The figure shows three views and two pictorial views of one solid part (mm, origin at its lowest corner). Answer the questions. A direction names the side the tool comes from. Coordinates: 2 decimals unless noted, no trailing zeros. Write each loop counter-clockwise with the first axis right and the second up, starting at its lowest first coordinate (ties: lowest second). Pieces come first, ordered by that corner, then holes.
Item 1: Section B-B (y = 112.5) is taken. Give the vertices of the cut face in (x, z), then the cut area to 3 significant figures.
Item 2: A tool of negligible diameter and unlimited length cuts with its end or side. For the marked faces 1 and 2, from which of +Z, -Z, +X, -X, +Y, -Y can it reach the whole face along a straight path? Write none if from no direction.
Item 3: Straight lines are drawn through the part: probe 1 along Y at (x, z) = (17.5, 30); probe 2 along Z at (x, y) = (13.75, 136) (1 decimal); probe 3 along Z at (x, y) = (17.25, 158) (1 decimal). For each, find the intervals that lie inside material, in ascending order.
Item 4: Determine the mould class of the marked faces 3, 4 and 5 for opening direction Z: released by +Z, released by -Z, zero draft, split by the parting line, or undercut.
Item 5: Section A-A (y = 67) is taken. Give the vertices of the cut face in (x, z).
Item 6: Each of these flat-tipped pins is pushed along its axis until it touches: P1, Ø4, axis at x = 19, y = 20.5, coming from the -Z side; P2, Ø12, axis at x = 21, y = 142.5, coming from the +Z side; P3, Ø5, axis at x = 12.5, y = 91.5, coming from the -Z side; P4, Ø5, axis at x = 8, z = 6, coming from the -Y side. Where does it stop, or does it pass through?
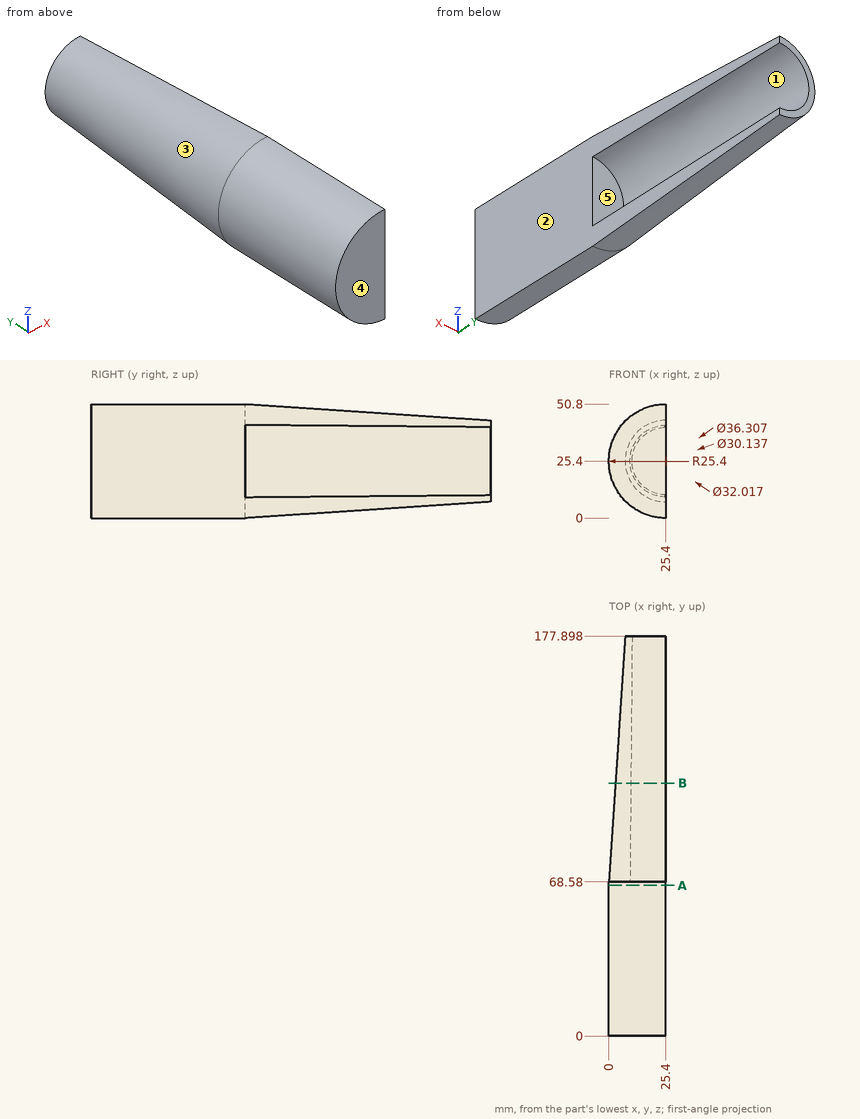
Established:
1. outline: (25.4, 2.91) - (25.4, 9.77) arc R15.63 cw to (25.4, 41.03) - (25.4, 47.89) arc R22.49 ccw to start
1. area: 411 mm2
2. face 1: +X
2. face 2: +Z, -Z, +X, +Y, -Y
3. probe 1: y = 0 to 68.58
3. probe 2: z = 8 to 15.3, 35.5 to 42.8
3. probe 3: z = 7.7 to 12.5, 38.3 to 43.1
4. face 3: split by the parting line
4. face 4: zero draft
4. face 5: undercut
5. outline: (25.4, 0) - (25.4, 50.8) arc R25.4 ccw to start
6. P1: stops at z = 0.38
6. P2: stops at z = 46.2
6. P3: stops at z = 3.89
6. P4: stops at y = 0
